The listing builds one solid part. Answer for the finished solid, in the listing's coordinates (mm). Round coordinates to 2 decimals unless told otherwise and drop trailing zeros. Write each loop counter-clockwise with the first axis right and the second up, starting at its lowest first coordinate (ties: lowest second). Pieces come first, ordered by that corner, then holes. Notation, with made-up numbers: M 82.5,20 L 113.5,20 A29 cw 113.5,45 Z; hole C 24.5,59 d4. An arc over 180 degrees is marked long. Put each result on its own line as item: value. Start each with the question number.
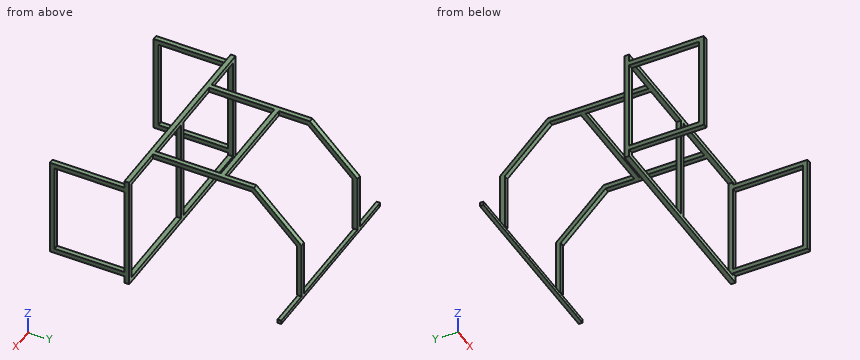
```python
from build123d import *

# Parameters (mm, degrees)
SKETCH1_W           = 1074.6
SKETCH1_H           = 620
SKETCH1_W_2         = 1023.8
SKETCH1_H_2         = 569.2
BOSS_EXTRUDE1_DEPTH = 25.4
SKETCH2_W           = 25.4
SKETCH2_H           = 25.4
BOSS_EXTRUDE2_DEPTH = 400
SKETCH3_W           = 25.4
SKETCH3_H           = 25.4
BOSS_EXTRUDE3_DEPTH = 490.4
SKETCH5_W           = 25.4
SKETCH5_H           = 25.4
BOSS_EXTRUDE5_DEPTH = 50
SKETCH4_W           = 25.4
SKETCH4_H           = 569.2
BOSS_EXTRUDE6_DEPTH = 25.4
BOSS_EXTRUDE7_DEPTH = 25.4
SKETCH9_W           = 25.4
SKETCH9_H           = 25.4
BOSS_EXTRUDE8_DEPTH = 270
SKETCH10_W          = 1000
SKETCH10_H          = 20
BOSS_EXTRUDE9_DEPTH = 20


with BuildPart() as part:
    # Sketch1 → Boss-Extrude1 (new body)
    with BuildSketch(Plane(origin=(0, 0, 0), x_dir=(1, 0, 0), z_dir=(0, 1, 0))):
        Rectangle(SKETCH1_W, SKETCH1_H)
        Rectangle(SKETCH1_W_2, SKETCH1_H_2, mode=Mode.SUBTRACT)
    extrude(amount=BOSS_EXTRUDE1_DEPTH)

    # Sketch2 → Boss-Extrude2 (add)
    with BuildSketch(Plane.XZ):
        with Locations((-524.6, 257.9)):
            Rectangle(SKETCH2_W, SKETCH2_H)
        with Locations((-524.6, -257.9)):
            Rectangle(SKETCH2_W, SKETCH2_H)
        with Locations((524.6, 257.9)):
            Rectangle(SKETCH2_W, SKETCH2_H)
        with Locations((524.6, -257.9)):
            Rectangle(SKETCH2_W, SKETCH2_H)
    extrude(amount=BOSS_EXTRUDE2_DEPTH)

    # Sketch3 → Boss-Extrude3 (add)
    with BuildSketch(Plane(origin=(0, 0, 245.2), x_dir=(-1, 0, 0), z_dir=(0, 0, -1))):
        with Locations((524.6, -387.3)):
            Rectangle(SKETCH3_W, SKETCH3_H)
        with Locations((-524.6, -387.3)):
            Rectangle(SKETCH3_W, SKETCH3_H)
    extrude(amount=BOSS_EXTRUDE3_DEPTH)

    # Sketch5 → Boss-Extrude5 (add)
    with BuildSketch(Plane(origin=(0, 25.4, 0), x_dir=(1, 0, 0), z_dir=(0, 1, 0))):
        with Locations((282.7, -297.3)):
            Rectangle(SKETCH5_W, SKETCH5_H)
    boss_extrude5 = extrude(amount=BOSS_EXTRUDE5_DEPTH)

    # Sketch4 → Boss-Extrude6 (add)
    with BuildSketch(Plane(origin=(0, 25.4, 0), x_dir=(1, 0, 0), z_dir=(0, 1, 0))):
        Rectangle(SKETCH4_W, SKETCH4_H)
    extrude(amount=-BOSS_EXTRUDE6_DEPTH)

    # Sketch8 → Boss-Extrude7 (add)
    with BuildSketch(Plane(origin=(295.4, 0, 0), x_dir=(0, 0, -1), z_dir=(1, 0, 0))):
        Polygon((-284.6, 75.4), (-284.6, 555.4), (-44.6, 795.4), (255.4, 795.4), (255.4, 820.8), (-55.121024484, 820.8), (-310, 565.921024484), (-310, 75.4), align=None)
    boss_extrude7 = extrude(amount=-BOSS_EXTRUDE7_DEPTH)

    # Sketch9 → Boss-Extrude8 (add)
    with BuildSketch(Plane.ZY.offset(-270)):
        with Locations((297.3, 388.1)):
            Rectangle(SKETCH9_W, SKETCH9_H)
    boss_extrude8 = extrude(amount=BOSS_EXTRUDE8_DEPTH)

    # Mirror1: Boss-Extrude5, Boss-Extrude7, Boss-Extrude8 across plane
    add(boss_extrude5.mirror(Plane.ZY))
    add(boss_extrude7.mirror(Plane.ZY))
    add(boss_extrude8.mirror(Plane.ZY))

    # Sketch10 → Boss-Extrude9 (add)
    with BuildSketch(Plane(origin=(0, 820.8, 0), x_dir=(1, 0, 0), z_dir=(0, 1, 0))):
        with Locations((0, 265.4)):
            Rectangle(SKETCH10_W, SKETCH10_H)
    extrude(amount=-BOSS_EXTRUDE9_DEPTH)


solid = part.part
```
Item 1: Section C-C (z = -127) is taken. Give the vertices of the cut face in (x, y).
Item 2: Flat-ended cylindrical pins translate along their axes: pin 1 (6 mm diameter, centred on x = -74, z = -266.5, fed in from -Y); pin 2 (16 mm diameter, centred on x = 368, y = 810, fed in from +Z); pin 3 (7.5 mm diameter, centred on x = 521.5, z = -55.5, fed in from +Y). Find the tip coordinate at first contact, or state that the pin passes through.
Item 3: Section B-B (x = 57.5) is taken. Give the vertices of the cut face in (y, z).
Item 4: Section D-D (x = -460) is taken. Give the vertices of the cut face in (y, z).
Item 5: Consider line 1 along Y through (x, z) = (200.5, -255.5); line 2 along Z through (x, y) = (122, 395). Determine where each line is inside the solid, lowest interval first. Write a range as [from, to].
Item 6: Section A-A (y = -251) is taken. Give the vertices of the cut face in (x, z).
Output values:
1. outline: M -537.3,-400 L -511.9,-400 L -511.9,-374.6 L -537.3,-374.6 Z; M -537.3,0 L -511.9,0 L -511.9,25.4 L -537.3,25.4 Z; M -295.4,795.4 L -270,795.4 L -270,820.8 L -295.4,820.8 Z; M -12.7,0 L 12.7,0 L 12.7,25.4 L -12.7,25.4 Z; M 270,795.4 L 295.4,795.4 L 295.4,820.8 L 270,820.8 Z; M 511.9,-400 L 537.3,-400 L 537.3,-374.6 L 511.9,-374.6 Z; M 511.9,0 L 537.3,0 L 537.3,25.4 L 511.9,25.4 Z
2. pin 1: stops at y = 800.8
2. pin 2: stops at z = -255.4
2. pin 3: stops at y = 25.4
3. outline: M 0,-310 L 25.4,-310 L 25.4,-284.6 L 0,-284.6 Z; M 0,284.6 L 25.4,284.6 L 25.4,310 L 0,310 Z; M 375.4,284.6 L 400.8,284.6 L 400.8,310 L 375.4,310 Z; M 800.8,-275.4 L 820.8,-275.4 L 820.8,-255.4 L 800.8,-255.4 Z
4. outline: M 0,-310 L 25.4,-310 L 25.4,-284.6 L 0,-284.6 Z; M 0,284.6 L 25.4,284.6 L 25.4,310 L 0,310 Z; M 800.8,-275.4 L 820.8,-275.4 L 820.8,-255.4 L 800.8,-255.4 Z
5. line 1: y = [800.8, 820.8]
5. line 2: z = [284.6, 310]
6. outline: M -537.3,-270.6 L -511.9,-270.6 L -511.9,-245.2 L -537.3,-245.2 Z; M -537.3,245.2 L -511.9,245.2 L -511.9,270.6 L -537.3,270.6 Z; M 511.9,-270.6 L 537.3,-270.6 L 537.3,-245.2 L 511.9,-245.2 Z; M 511.9,245.2 L 537.3,245.2 L 537.3,270.6 L 511.9,270.6 Z
